Read the model definition and answer for the solid it produces. Units are mm, in the model's axes. A direction names the side the tool comes from. Give positions to 0.01 mm unless a question says otherwise; leave off trailing zeros. Write each loop counter-clockwise with the first axis right and the second up, starting at its lowest first coordinate (ties: lowest second). Pieces come first, ordered by that corner, then holes. Notation, with made-up numbers: M -39,85 L 10,85 A22 ccw 10,101 Z; hole C -8.5,-18 d2. An arc over 180 degrees is marked long. Use a Markdown table: item, result. Add a question column.
Item 1: The mould has two halves that part along Y. Classify faces 1 (the flat face through (44, 25, 2)), 2 (the flat face through (93.742, 0, 2)), 3 (the flat face through (-97, -10.001, 2)), 4 (the flat face through (-1, -25, 2)): pulls with the +Y half, pulls with the -Y half, needs draft (parallel to the pull), parting line crosses it, or undercut.
Item 2: For faces 5 (the flat face through (93.742, -29, 2)), 6 (the flat face through (-94.258, -29, 2)), 7 (the flat face through (96, -10.001, 2)), 8 (the flat face through (73, 20, 2)), determine the directions among +Z, -Z, +X, -X, +Y, -Y from which every point of the face is accessible in a straight line to the end or side of a thin tool.
Item 3: Consider probe 1 along X at (y, z) = (-28.5, 0.6); probe 2 along Y at (x, z) = (0, 2); probe 3 along Y at (x, z) = (-4, 1.75). Determine where each line is inside the solid, lowest interval first. Write a range as [from, to].
Item 4: A cutting plane is placed at B-B on y = 0. Determine the outline of the cut face in (x, z), then the cut area to 3 significant figures.
Item 5: A cutting plane is placed at C-C on y = 7.5. Determine the outline of the cut face in (x, z), then the cut area to 3 significant figures.
Item 6: Given P1, Ø2, axis at y = 6, z = 3, coming from the +X side; P2, Ø1.5, axis at x = -97.5, z = 1.5, coming from the -Y side; P3, Ø2.5, axis at x = 0, y = 0, coming from the +Z side; P4, Ø2.5, axis at y = -31, z = 3, coming from the -X side, each flat-ended and moving along its own axis, determine where each tip first touches the part or whether it passes through.
Item 7: A cutting plane is placed at A-A on x = 0. Determine the outline of the cut face in (y, z), then the cut area to 3 significant figures.
Autodesk Inventor part; units mm, degrees
ref_plane "YZ Plane" through (0, 0, 0) normal (1, 0, 0) x (0, 1, 0)
ref_plane "XZ Plane" through (0, 0, 0) normal (0, 1, 0) x (-1, 0, 0)
ref_plane "XY Plane" through (0, 0, 0) normal (0, 0, 1) x (1, 0, 0)
sketch "Sketch1" plane through (0, 0, 0) normal (0, 0, 1) x (1, 0, 0)
  line L0 (-89.2581, -25.0004) -> (-89.2581, -33.0004)
  line L1 (-89.2581, -25.0004) -> (-58.0081, -25.0004)
  line L2 (-58.0081, -25.0004) -> (-58.0081, -33.0004)
  line L3 (-31.7581, -25.0004) -> (-31.7581, -33.0004)
  line L4 (-31.7581, -25.0004) -> (31.2419, -25.0004)
  line L5 (31.2419, -25.0004) -> (31.2419, -33.0004)
  line L6 (93.7419, -25.0004) -> (98.7419, -25.0004)
  line L7 (98.7419, -25.0004) -> (98.7419, -10.0012)
  line L8 (93.7419, -10.0012) -> (98.7419, -10.0012)
  line L9 (93.7419, -10.0012) -> (93.7419, 9.9988)
  line L10 (93.7419, 9.9988) -> (98.7419, 9.9988)
  line L11 (98.7419, 9.9988) -> (98.7419, 25.0003)
  line L12 (-99.2581, 9.9988) -> (-99.2581, 25.0003)
  line L13 (-99.2581, 9.9988) -> (-94.2581, 9.9988)
  line L14 (-99.2581, -10.0012) -> (-99.2581, -25.0004)
  line L15 (-99.2581, -10.0012) -> (-94.2581, -10.0012)
  line L16 (-99.2581, -25.0004) -> (-94.2581, -25.0004)
  line L17 (-94.2581, 9.9988) -> (-94.2581, -10.0012)
  line L18 (-94.2581, -25.0004) -> (-94.2581, -33.0004)
  line L19 (93.7419, -33.0004) -> (93.7419, -25.0004)
  line L20 (-89.2581, 25.0003) -> (-89.2581, 20.0003)
  line L21 (-89.2581, 20.0003) -> (-58.0081, 20.0003)
  line L22 (-58.0081, 25.0003) -> (-58.0081, 20.0003)
  line L23 (-58.0081, 25.0003) -> (-31.7581, 25.0003)
  line L24 (-31.7581, 25.0003) -> (-31.7581, 20.0003)
  line L25 (-31.7581, 20.0003) -> (31.2419, 20.0003)
  line L26 (31.2419, 25.0003) -> (31.2419, 20.0003)
  line L27 (31.2419, 25.0003) -> (57.4919, 25.0003)
  line L28 (57.4919, 25.0003) -> (57.4919, 20.0003)
  line L29 (57.4919, 20.0003) -> (88.7419, 20.0003)
  line L30 (88.7419, 25.0003) -> (88.7419, 20.0003)
  line L31 (-89.2581, 25.0003) -> (-99.2581, 25.0003)
  line L32 (88.7419, 25.0003) -> (98.7419, 25.0003)
  circle A0 centre (0, 0) radius 2
  line L33 (57.4919, -33.0004) -> (57.4919, -25.0004)
  line L34 (57.4919, -25.0004) -> (88.7419, -25.0004)
  line L35 (88.7419, -25.0004) -> (88.7419, -33.0004)
  line L36 (88.7419, -33.0004) -> (93.7419, -33.0004)
  line L37 (31.2419, -33.0004) -> (57.4919, -33.0004)
  line L38 (-94.2581, -33.0004) -> (-89.2581, -33.0004)
  line L39 (-58.0081, -33.0004) -> (-31.7581, -33.0004)
  point P0 (-93.0453, -16.9364)
  dimension "d46" = 198
  dimension "d47" = 4
  dimension "d48" = 26.25
  dimension "d50" = 63
  dimension "d51" = 31.25
  dimension "d56" = 45.0007
  dimension "d57" = 50.0007
  dimension "d59" = 5
extrude "Extrusion3" add sketch "Sketch1" along normal blind 5
properties part number "case bottom sides" material "ABS Plastic"
Filled in:
| question | item | result |
|---|---|---|
| 1 | face 1 | pulls with the +Y half |
| 1 | face 2 | undercut |
| 1 | face 3 | undercut |
| 1 | face 4 | pulls with the -Y half |
| 2 | face 5 | +Z, -Z, +X, -Y |
| 2 | face 6 | +Z, -Z, -X, -Y |
| 2 | face 7 | +Z, -Z, +X |
| 2 | face 8 | +Z, -Z, +Y |
| 3 | probe 1 | [-94.26, -89.26], [-58.01, -31.76], [31.24, 57.49], [88.74, 93.74] |
| 3 | probe 2 | [-25, -2], [2, 20] |
| 3 | probe 3 | [-25, 20] |
| 4 | outline | M -94.26,0 L -2,0 L -2,5 L -94.26,5 Z; M 2,0 L 93.74,0 L 93.74,5 L 2,5 Z |
| 4 | area | 920 mm² |
| 5 | outline | M -94.26,0 L 93.74,0 L 93.74,5 L -94.26,5 Z |
| 5 | area | 940 mm² |
| 6 | P1 | x = 93.74 |
| 6 | P2 | y = -25 |
| 6 | P3 | through |
| 6 | P4 | x = -94.26 |
| 7 | outline | M -25,0 L -2,0 L -2,5 L -25,5 Z; M 2,0 L 20,0 L 20,5 L 2,5 Z |
| 7 | area | 205 mm² |
